```python
from build123d import *

# Parameters (mm, degrees)
SKETCH1_R                      = 12.5
BOSS_EXTRUDE1_DEPTH            = 20
SKETCH2_W                      = 90
SKETCH2_H                      = 60
BOSS_EXTRUDE2_DEPTH            = 90
SKETCH6_W                      = 60
SKETCH6_H                      = 100
BOSS_EXTRUDE4_DEPTH            = 400
SKETCH8_W                      = 120
SKETCH8_H                      = 340
CUT_EXTRUDE4_DEPTH             = 507.384241461
BOSS_EXTRUDE5_DEPTH            = 30
BOSS_EXTRUDE6_START            = -30
BOSS_EXTRUDE6_DEPTH            = 30
CUT_EXTRUDE6_DEPTH             = 180
SKETCH12_W                     = 50
SKETCH12_H                     = 80
BOSS_EXTRUDE7_DEPTH            = 50
SKETCH14_W                     = 40
SKETCH14_H                     = 100
BOSS_EXTRUDE8_DEPTH            = 50
SKETCH13_R                     = 12.5
CUT_EXTRUDE7_DEPTH             = 100
CUT_EXTRUDE7_DIRECTION_2_REACH = 533.272


with BuildPart() as part:
    # Sketch1 → Boss-Extrude1 (new body)
    with BuildSketch(Plane(origin=(0, 0, 0), x_dir=(0, 0, -1), z_dir=(1, 0, 0))):
        Circle(SKETCH1_R)
    extrude(amount=BOSS_EXTRUDE1_DEPTH)

    # Sketch2 → Boss-Extrude2 (add)
    with BuildSketch(Plane(origin=(20, 0, 0), x_dir=(0, 0, -1), z_dir=(1, 0, 0))):
        Rectangle(SKETCH2_W, SKETCH2_H)
    extrude(amount=BOSS_EXTRUDE2_DEPTH)

    # Mirror1: part across plane


with BuildPart() as part_1:
    add(part.part)
    add(part.part.mirror(Plane.ZY.offset(-110)))

    # Sketch6 → Boss-Extrude4 (add)
    with BuildSketch(Plane(origin=(0, 0, -45), x_dir=(-1, 0, 0), z_dir=(0, 0, -1))):
        with Locations((-50, 0)):
            Rectangle(SKETCH6_W, SKETCH6_H)
        with Locations((-170, 0)):
            Rectangle(SKETCH6_W, SKETCH6_H)
    extrude(amount=BOSS_EXTRUDE4_DEPTH)

    # Sketch8 → Cut-Extrude4 (cut, through all)
    with BuildSketch(Plane(origin=(0, 50, 0), x_dir=(1, 0, 0), z_dir=(0, 1, 0))):
        with Locations((110, 275)):
            Rectangle(SKETCH8_W, SKETCH8_H)
    extrude(amount=-CUT_EXTRUDE4_DEPTH, mode=Mode.SUBTRACT)

    # Sketch9 → Boss-Extrude5 (add)
    with BuildSketch(Plane.ZY.offset(-20)):
        Polygon((-445, 50), (-245, 100), (-45, 50), align=None)
    extrude(amount=-BOSS_EXTRUDE5_DEPTH)

    # Sketch10 → Boss-Extrude6 (add)
    with BuildSketch(Plane(origin=(200, 0, 0), x_dir=(0, 0, -1), z_dir=(1, 0, 0)).offset(BOSS_EXTRUDE6_START)):
        Polygon((245, 100), (445, 50), (45, 50), align=None)
    extrude(amount=BOSS_EXTRUDE6_DEPTH)

    # Sketch11 → Cut-Extrude6 (cut)
    with BuildSketch(Plane(origin=(200, 0, 0), x_dir=(0, 0, -1), z_dir=(1, 0, 0))):
        Polygon((70.294812967, 6.954060935), (106.010734034, 41.166153746), (70.294812967, 41.166153746), align=None)
        Polygon((70.294812967, -27.258031877), (141.726655101, -27.258031877), (141.726655101, 41.166153746), align=None)
        Polygon((186.841502765, 64.475491706), (228.19677979, 64.475491706), (186.841502765, -27.258031877), align=None)
        Polygon((228.19677979, -27.258031877), (269.552056815, -27.258031877), (269.552056815, 18.608729914), align=None)
        Polygon((313.914990351, 41.166153746), (348.87899729, 41.166153746), (313.914990351, 6.954060935), align=None)
        Polygon((313.914990351, -27.258031877), (383.843004229, -27.258031877), (383.843004229, 6.954060935), align=None)
    extrude(amount=-CUT_EXTRUDE6_DEPTH, mode=Mode.SUBTRACT)

    # Sketch12 → Boss-Extrude7 (add)
    with BuildSketch(Plane(origin=(0, 0, -445), x_dir=(-1, 0, 0), z_dir=(0, 0, -1))):
        with Locations((-35, 0)):
            Rectangle(SKETCH12_W, SKETCH12_H)
    extrude(amount=BOSS_EXTRUDE7_DEPTH)

    # Sketch14 → Boss-Extrude8 (add, through all)
    with BuildSketch(Plane(origin=(0, 0, -445), x_dir=(-1, 0, 0), z_dir=(0, 0, -1))):
        with Locations((-205, 0)):
            Rectangle(SKETCH14_W, SKETCH14_H)
    extrude(amount=BOSS_EXTRUDE8_DEPTH)

    # Sketch13 → Cut-Extrude7 (cut)
    with BuildSketch(Plane(origin=(60, 0, 0), x_dir=(0, 0, -1), z_dir=(1, 0, 0))):
        with Locations(Location((470, 0, 0), (0, 0, 180))):
            Circle(SKETCH13_R)
    extrude(amount=-CUT_EXTRUDE7_DEPTH, mode=Mode.SUBTRACT)

    # Sketch13 → Cut-Extrude7 direction 2 (cut, up to next)
    with BuildSketch(Plane(origin=(60, 0, 0), x_dir=(0, 0, -1), z_dir=(1, 0, 0)), mode=Mode.PRIVATE) as cut_extrude7_direction_2_sk1:
        with Locations(Location((470, 0, 0), (0, 0, 180))):
            Circle(SKETCH13_R)
    cut_extrude7_direction_2_tool1 = extrude(cut_extrude7_direction_2_sk1.sketch, amount=CUT_EXTRUDE7_DIRECTION_2_REACH, mode=Mode.PRIVATE) & part_1.part
    add(cut_extrude7_direction_2_tool1.solids().sort_by_distance((60, 0, -470))[0], mode=Mode.SUBTRACT)


solid = part_1.part
```
For this review, take the finished solid that the model builds, in its own axes (mm). A direction names the side the tool comes from. Round coordinates to 2 decimals unless told otherwise and drop trailing zeros. Write each loop counter-clockwise with the first axis right and the second up, starting at its lowest first coordinate (ties: lowest second). Pieces come first, ordered by that corner, then holes.
1) For line 1 along X through (y, z) = (9, -73); line 2 along X through (y, z) = (-42, -432); line 3 along Z through (x, y) = (52, -39), list the stretches that pass through material, from the lowest coordinate up.
Answer below:
line 1: x = 20 to 80, 140 to 200
line 2: x = 20 to 50, 170 to 200
line 3: z = -495 to -445, -105 to -45
2) Insertion check: pin 1 Ø6 at (x, y) = (51, 39.5) entering from +Z; pin 2 Ø8 at (x, y) = (167, 43.5) entering from -Z; pin 3 Ø15 at (y, z) = (-20, -478.5) entering from -X. Each pin has a flat end and moves straight along its axis. Give the tip position at first contact, or say it passes through.
Answer below:
pin 1: stops at z = -45
pin 2: stops at z = -445
pin 3: stops at x = 10
3) Take a section at B-B on y = 71.5. Give the boundary of the cut face in (x, z), then the cut area to 3 significant figures.
Answer below:
outline: (20, -359) - (50, -359) - (50, -131) - (20, -131) - close; (170, -359) - (200, -359) - (200, -131) - (170, -131) - close
area: 13,700 mm2
4) Take a section at A-A on z = -392. Give the boundary of the cut face in (x, y), then the cut area to 4 significant figures.
Answer below:
outline: (20, -50) - (50, -50) - (50, 63.25) - (20, 63.25) - close; (170, -50) - (200, -50) - (200, 63.25) - (170, 63.25) - close
area: 6,795 mm2
5) Take a section at C-C on x = 40. State how many separate pieces and enclosed holes the cut face has, then the cut area to 3 significant figures.
Answer below:
separate pieces: 1
enclosed holes: 7
area: 51,200 mm2
6) Take a section at D-D on z = -470. Give the boundary of the cut face in (x, y).
Answer below:
outline: (10, -40) - (60, -40) - (60, -12.5) - (10, -12.5) - close; (10, 12.5) - (60, 12.5) - (60, 40) - (10, 40) - close; (185, -50) - (225, -50) - (225, -12.5) - (185, -12.5) - close; (185, 12.5) - (225, 12.5) - (225, 50) - (185, 50) - close
7) Mouldability with a two-part tool opening along Z and no side actions: class faces 4 (the face through (200, -7, -203)), 5 (the face through (34.79, 75.35, -146.4)), 6 (the face through (34.79, 74.65, -346.4)) as +Z half, -Z half, draft (parallel to the pull), parting line (faces both ways), or undercut.
Answer below:
face 4: undercut
face 5: +Z half
face 6: -Z half
8) Machinability: for faces 1 (the face through (35.21, 24.3, -331.64)), 2 (the face through (35, 40, -470)), 3 (the face through (170, -40, -45)), which of the approach directions +Z, -Z, +X, -X, +Y, -Y give a long, thin tool a straight path to every point of the face, cutting with its end or side? Answer none if there is none.
Answer below:
face 1: +X, -X
face 2: -Z, -X, +Y
face 3: +Z, +X, -X, -Y
